For this review, use the dimensioned drawing (mm, ordinates from the lowest corner) and the shaded views. A direction names the side the tool comes from. Coordinates: 2 decimals unless noted, no trailing zeros. Write each loop counter-clockwise with the first axis right and the second up, starting at its lowest first coordinate (ties: lowest second). Pieces come first, ordered by that corner, then holes. Notation, with made-up numbers: M 57,-25 L 61,-25 A9 cw 61,-8 Z; hole C 53.25,32 d6. An arc over 180 degrees is marked long. One line per question, with ' | ' between items.
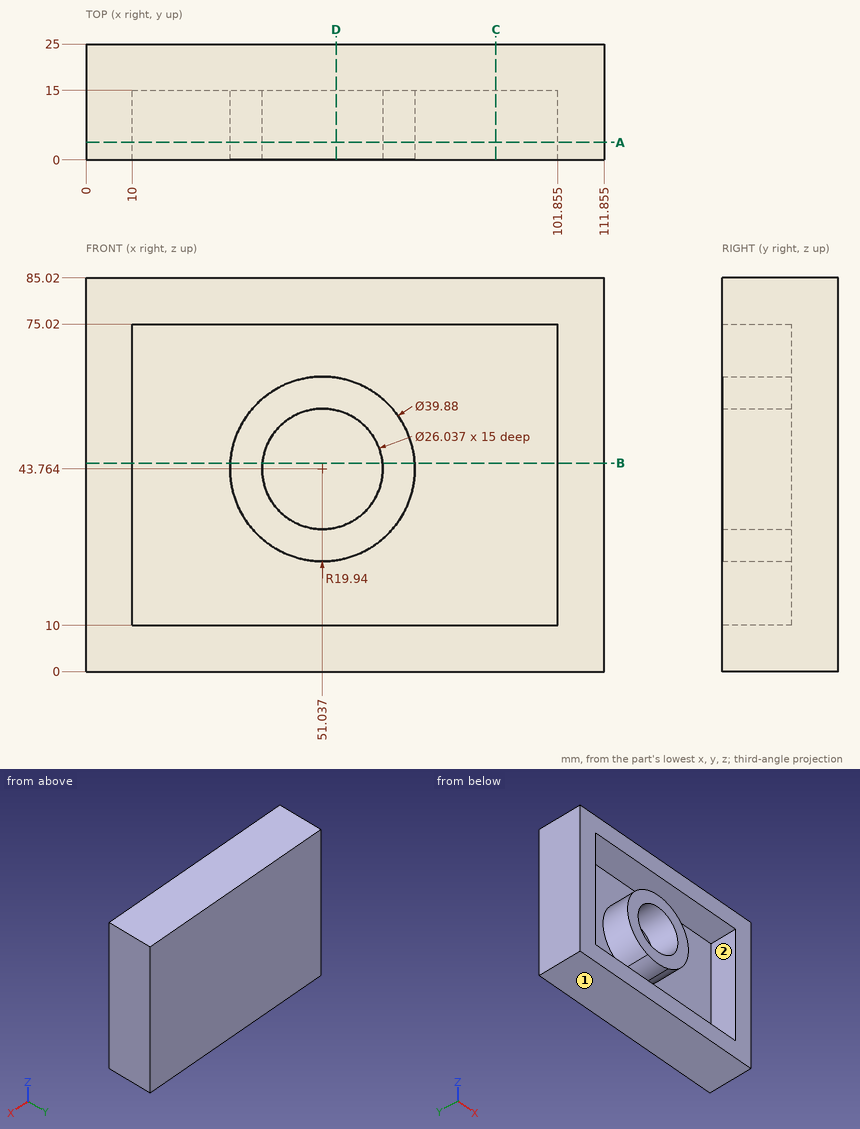
1) We need section B-B on z = 45. State the section outline as (x, y) points (1 decimal).
Responses:
outline: M 0,0 L 10,0 L 10,15 L 31.1,15 L 31.1,0 L 38.1,0 L 38.1,15 L 64,15 L 64,0 L 70.9,0 L 70.9,15 L 101.9,15 L 101.9,0 L 111.9,0 L 111.9,25 L 0,25 Z
2) Insertion check: pin 1 Ø7.5 at (y, z) = (8, 35.5) entering from -X; pin 2 Ø23.5 at (x, z) = (51.04, 43.76) entering from -Y. Each pin has a flat end and moves straight along its axis. Give the tip position at first contact, or say it passes through.
Responses:
pin 1: x = 0 | pin 2: y = 15
3) We need section C-C on x = 88.5. State the section outline as (y, z) points.
Responses:
outline: M 0,0 L 25,0 L 25,85.02 L 0,85.02 L 0,75.02 L 15,75.02 L 15,10 L 0,10 Z
4) Machinability: for the marked faces 1 and 2, which of the approach directions +Z, -Z, +X, -X, +Y, -Y give a long, thin tool a straight path to every point of the face, cutting with its end or side? Answer none if there is none.
Responses:
face 1: -Z, +X, -X, +Y, -Y | face 2: -Y
5) To check wall thickness, follow line 1 along Z through (x, y) = (60, 14.25) (1 decimal); line 2 along Z through (x, y) = (81.5, 8.25); line 3 along X through (y, z) = (10.75, 46.5) (1 decimal). State the ranges of each line that lie inside material, in increasing order. Write a range as [from, to].
Responses:
line 1: [0, 10], [26, 34.3], [53.2, 61.6], [75, 85] | line 2: [0, 10], [75.02, 85.02] | line 3: [0, 10], [31.3, 38.3], [63.8, 70.8], [101.9, 111.9]
6) We need section D-D on x = 54. State the section outline as (y, z) points (1 decimal), then the cut area to 3 significant figures.
Responses:
outline: M 0,0 L 25,0 L 25,85 L 0,85 L 0,75 L 15,75 L 15,63.5 L 0,63.5 L 0,56.4 L 15,56.4 L 15,31.1 L 0,31.1 L 0,24 L 15,24 L 15,10 L 0,10 Z | area: 1,360 mm^2
7) We need section A-A on y = 3.75. State the section outline as (x, z) points (1 decimal).
Responses:
outline: M 0,0 L 111.9,0 L 111.9,85 L 0,85 Z; M 44.3,25 A19.9 ccw 57.8,25 A19.9 ccw 71,43.8 A19.9 ccw long Z; hole M 10,10 L 101.9,10 L 101.9,75 L 10,75 Z; hole C 51,43.8 d26
